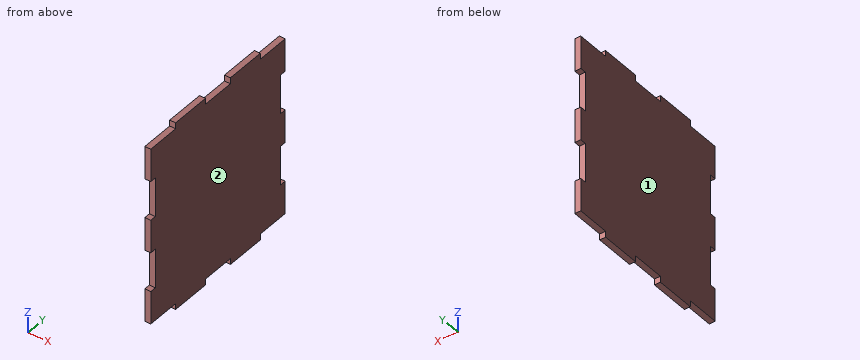
from build123d import *

# Parameters (mm, degrees)
F0_W     = 20
F0_H     = 3.05
F1_DEPTH = 3


# Not quite as in the source:
# - a feature names something its author has since deleted; it is built from what else it names


with BuildPart() as f1:
    # F0 (on Right) → F1 (new body)
    with BuildSketch(Plane.YZ):
        Polygon((28.35, -45), (45, -45), (45, -28.3), (41.95, -28.3), (41.95, -8.4), (45, -8.4), (45, 8.4), (41.95, 8.4), (41.95, 28.3), (45, 28.3), (45, 45), (28.35, 45), (8.35, 45), (-8.35, 45), (-28.35, 45), (-45, 45), (-45, 28.3), (-41.95, 28.3), (-41.95, 8.4), (-45, 8.4), (-45, -8.4), (-41.95, -8.4), (-41.95, -28.3), (-45, -28.3), (-45, -45), (-28.35, -45), (-8.35, -45), (8.35, -45), align=None)
        with Locations((-18.35, -46.525)):
            Rectangle(F0_W, F0_H)
        with Locations((18.35, -46.525)):
            Rectangle(F0_W, F0_H)
        with Locations((18.35, 46.525)):
            Rectangle(F0_W, F0_H)
        with Locations((-18.35, 46.525)):
            Rectangle(F0_W, F0_H)
    extrude(amount=F1_DEPTH)


solid = f1.part
Here's how the part is built. I have some questions about the finished solid (model axes, mm). Face numbers are marked on the shaded views. Round coordinates to 2 decimals unless told otherwise and drop trailing zeros. Loops run counter-clockwise (first coordinate to the right, second up) from the corner with the lowest first, then second, coordinate; pieces in that order, holes last. Notation, with made-up numbers: (61, 84) -> (111, 84) arc R16 ccw to (111, 115) -> close; hole circle Ø2 at (23.5, -14). An arc over 180 degrees is marked (long way). Write each question's results on one line, items separated by ' | '.
(1) If I drill on L1, parallel to Z at x = 1.45, y = 31.5; L2, parallel to Y at x = 0.3, z = 25, over which ranges is the centre line in solid material (lowest first)?
Worked answers:
L1: -45 to 45 | L2: -41.95 to 41.95
(2) We'd pull the mould along X, two halves only. Please class the marked faces 1 and 2: released by +X, released by -X, zero draft, split by the parting line, or undercut.
Worked answers:
face 1: released by -X | face 2: released by +X
(3) If we section it at B-B, the plane y = -35.5: List the corners of the cut face in (x, z) for me.
Worked answers:
outline: (0, -45) -> (3, -45) -> (3, 45) -> (0, 45) -> close
(4) If we section it at A-A, the plane z = 18.5: List the corners of the cut face in (x, y) for me.
Worked answers:
outline: (0, -41.95) -> (3, -41.95) -> (3, 41.95) -> (0, 41.95) -> close
(5) For P1, Ø1.5, axis at x = 2.5, y = 33.5, coming from the -Z side; P2, Ø1.5, axis at x = 1.5, y = -1, coming from the +Z side; P3, Ø0.9, axis at x = 2, z = -16, coming from the +Y side, each with a flat end and sliding along its axis, tell me the tip position at first contact or that it passes through.
Worked answers:
P1: z = -45 | P2: z = 45 | P3: y = 41.95
